Design review of the part shown in the three views and the two pictorial views. Dimensions are in mm from the part's minimum x, y and z. Give positions to 0.01 mm unless a question says otherwise; leave off trailing zeros. Loops run counter-clockwise (first coordinate to the right, second up) from the corner with the lowest first, then second, coordinate; pieces in that order, holes last.
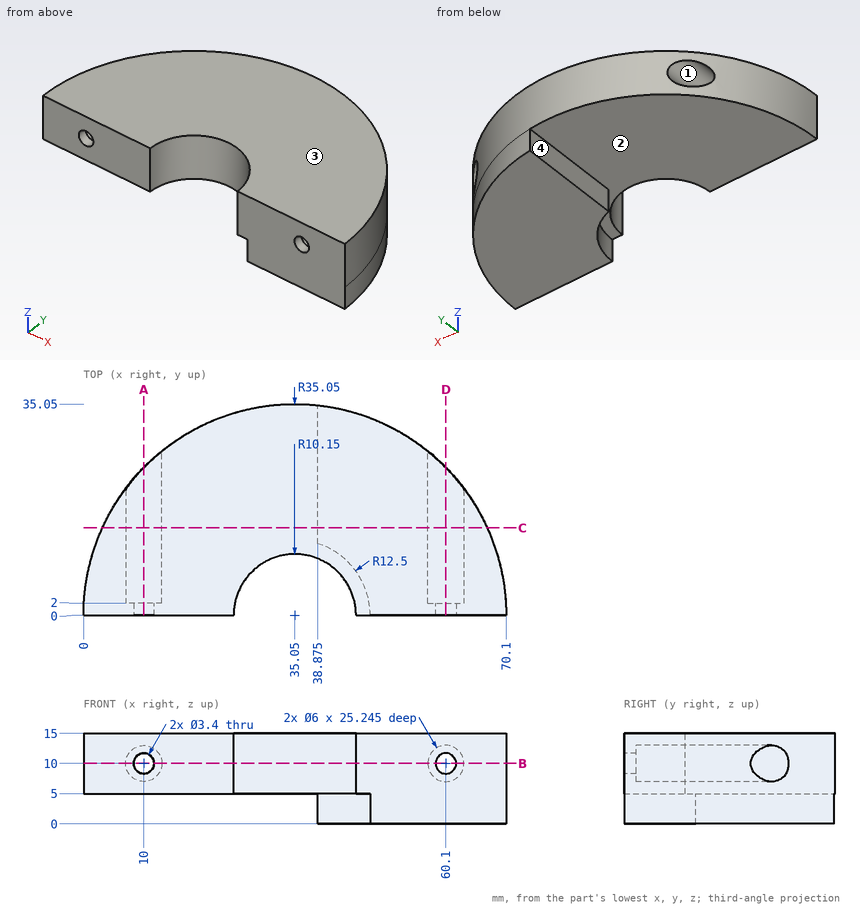
Q1. Mouldability with a two-part tool opening along Z and no side actions: class the marked faces 1, 2, 3 and 4 as +Z half, -Z half, draft (parallel to the pull), parting line (faces both ways), or undercut.
Answers:
face 1: undercut
face 2: -Z half
face 3: +Z half
face 4: draft
Q2. Consider section B-B on z = 10. Count the separate pieces of the cut face and the enclosed holes in it, plus the area to 3 significant figures.
Answers:
separate pieces: 3
enclosed holes: 0
area: 1,490 mm2
Q3. Consider section C-C on y = 14.5. Give the boundary of the cut face in (x, z) (3 decimals).
Answers:
outline: (3.14, 5) - (38.875, 5) - (38.875, 0) - (66.96, 0) - (66.96, 15) - (3.14, 15) - close; hole circle Ø6 at (10, 10); hole circle Ø6 at (60.1, 10)
Q4. For pin 1 Ø10.5 at (x, y) = (27.5, 17) entering from -Z; pin 2 Ø6.5 at (x, z) = (8.5, 9) entering from +Y (1 decimal); pin 3 Ø1.8 at (x, z) = (60, 10) entering from +Y; pin 4 Ø5.5 at (y, z) = (23.5, 2) entering from -X (3 decimals), all flat-tipped, find the tip position at first contact; note any pin that passes through.
Answers:
pin 1: stops at z = 5
pin 2: stops at y = 25.7
pin 3: passes through
pin 4: stops at x = 38.875
Q5. Consider section A-A on x = 10. Give the boundary of the cut face in (y, z) (1 decimal).
Answers:
outline: (0, 5) - (24.5, 5) - (24.5, 7) - (2, 7) - (2, 8.3) - (0, 8.3) - close; (0, 11.7) - (2, 11.7) - (2, 13) - (24.5, 13) - (24.5, 15) - (0, 15) - close
Q6. For probe 1 along X at (y, z) = (15.5, 10.5); probe 2 along X at (y, z) = (10.75, 10); probe 3 along X at (y, z) = (9, 10) (1 decimal), list the stretches that pass through material, from the lowest coordinate up.
Answers:
probe 1: x = 3.61 to 7.04, 12.96 to 57.14, 63.06 to 66.49
probe 2: x = 1.69 to 7, 13 to 57.1, 63.1 to 68.41
probe 3: x = 1.2 to 7, 13 to 30.4, 39.7 to 57.1, 63.1 to 68.9
Q7. Consider section D-D on x = 60.1. Give the boundary of the cut face in (y, z) (1 decimal).
Answers:
outline: (0, 0) - (24.5, 0) - (24.5, 7) - (2, 7) - (2, 8.3) - (0, 8.3) - close; (0, 11.7) - (2, 11.7) - (2, 13) - (24.5, 13) - (24.5, 15) - (0, 15) - close
